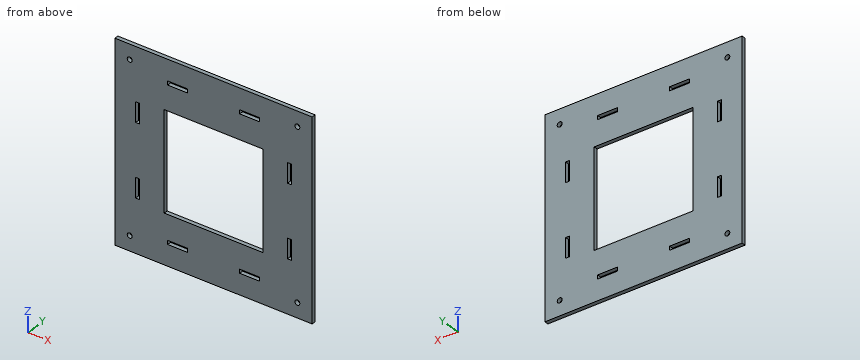
from build123d import *

# Parameters (mm, degrees)
CROQUIS1_W              = 200
CROQUIS1_H              = 200
CROQUIS1_R              = 2.5
SALIENTE_EXTRUIR1_DEPTH = 4
CROQUIS2_W              = 150
CROQUIS2_H              = 150
CROQUIS2_W_2            = 4
CROQUIS2_H_2            = 20
CROQUIS2_W_3            = 20
CROQUIS2_H_3            = 4
CORTAR_EXTRUIR1_DEPTH   = 4
CROQUIS3_W              = 150
CROQUIS3_H              = 150
CROQUIS3_W_2            = 100
CROQUIS3_H_2            = 100
SALIENTE_EXTRUIR2_DEPTH = 4


with BuildPart() as part:
    # Croquis1 → Saliente-Extruir1 (new body)
    with BuildSketch(Plane(origin=(0, 0, 0), x_dir=(1, 0, 0), z_dir=(0, 1, 0))):
        with Locations((100, 100)):
            Rectangle(CROQUIS1_W, CROQUIS1_H)
        with Locations(Location((15, 185, 0), (0, 0, 270))):
            Circle(CROQUIS1_R, mode=Mode.SUBTRACT)
        with Locations(Location((185, 185, 0), (0, 0, 270))):
            Circle(CROQUIS1_R, mode=Mode.SUBTRACT)
        with Locations(Location((185, 15, 0), (0, 0, 270))):
            Circle(CROQUIS1_R, mode=Mode.SUBTRACT)
        with Locations(Location((15, 15, 0), (0, 0, 270))):
            Circle(CROQUIS1_R, mode=Mode.SUBTRACT)
    extrude(amount=SALIENTE_EXTRUIR1_DEPTH)

    # Croquis2 → Cortar-Extruir1 (cut)
    with BuildSketch(Plane(origin=(0, 4, 0), x_dir=(1, 0, 0), z_dir=(0, 1, 0))):
        with Locations((100, 100)):
            Rectangle(CROQUIS2_W, CROQUIS2_H)
        with Locations((23, 136.5)):
            Rectangle(CROQUIS2_W_2, CROQUIS2_H_2)
        with Locations((63.5, 177)):
            Rectangle(CROQUIS2_W_3, CROQUIS2_H_3)
        with Locations((177, 136.5)):
            Rectangle(CROQUIS2_W_2, CROQUIS2_H_2)
        with Locations((136.5, 177)):
            Rectangle(CROQUIS2_W_3, CROQUIS2_H_3)
        with Locations((136.5, 23)):
            Rectangle(CROQUIS2_W_3, CROQUIS2_H_3)
        with Locations((177, 63.5)):
            Rectangle(CROQUIS2_W_2, CROQUIS2_H_2)
        with Locations((23, 63.5)):
            Rectangle(CROQUIS2_W_2, CROQUIS2_H_2)
        with Locations((63.5, 23)):
            Rectangle(CROQUIS2_W_3, CROQUIS2_H_3)
    extrude(amount=-CORTAR_EXTRUIR1_DEPTH, mode=Mode.SUBTRACT)

    # Croquis3 → Saliente-Extruir2 (add)
    with BuildSketch(Plane(origin=(0, 4, 0), x_dir=(1, 0, 0), z_dir=(0, 1, 0))):
        with Locations((100, 100)):
            Rectangle(CROQUIS3_W, CROQUIS3_H)
        with Locations((100, 100)):
            Rectangle(CROQUIS3_W_2, CROQUIS3_H_2, mode=Mode.SUBTRACT)
    extrude(amount=-SALIENTE_EXTRUIR2_DEPTH)


solid = part.part
The listing builds one solid part. Answer for the finished solid, in the listing's coordinates (mm). Round coordinates to 2 decimals unless told otherwise and drop trailing zeros. Order: outer loops, then holes, each group sorted by start corner. A loop starts at its lowest first (then second) coordinate and runs counter-clockwise, first axis right, second up. Notation, with made-up numbers: (32, 2.5) -> (47, 2.5) arc R28 ccw to (47, 28.5) -> close; hole circle Ø5 at (-13, 10.5). An arc over 180 degrees is marked (long way). One line per item, written item: value.
Item 1: Find section A-A, the plane z = -185. Give the vertices of the cut face in (x, y).
Taken from the geometry:
outline: (0, 0) -> (12.5, 0) -> (12.5, 4) -> (0, 4) -> close; (17.5, 0) -> (182.5, 0) -> (182.5, 4) -> (17.5, 4) -> close; (187.5, 0) -> (200, 0) -> (200, 4) -> (187.5, 4) -> close
Item 2: Straight lines are drawn through the part: L1, parallel to X at y = 2.8, z = -15; L2, parallel to X at y = 2.55, z = -176.5; L3, parallel to X at y = 2.1, z = -140. For each, find the intervals that lie inside material, in ascending order.
Taken from the geometry:
L1: x = 0 to 12.5, 17.5 to 182.5, 187.5 to 200
L2: x = 0 to 53.5, 73.5 to 126.5, 146.5 to 200
L3: x = 0 to 21, 25 to 50, 150 to 175, 179 to 200
Item 3: Find section C-C, the plane z = -124. Give the vertices of the cut face in (x, y), then the cut area to 3 significant figures.
Taken from the geometry:
outline: (0, 0) -> (50, 0) -> (50, 4) -> (0, 4) -> close; (150, 0) -> (200, 0) -> (200, 4) -> (150, 4) -> close
area: 400 mm2
Item 4: Find section D-D, the plane x = 15. Give the vertices of the cut face in (y, z).
Taken from the geometry:
outline: (0, -200) -> (4, -200) -> (4, -187.5) -> (0, -187.5) -> close; (0, -182.5) -> (4, -182.5) -> (4, -17.5) -> (0, -17.5) -> close; (0, -12.5) -> (4, -12.5) -> (4, 0) -> (0, 0) -> close
Item 5: Given P1, Ø3, axis at x = 15, z = -15, coming from the +Y side, flat-ended and moving along its own axis, determine where the tip first touches the part or whether it passes through.
Taken from the geometry:
P1: passes through
Item 6: Find section B-B, the plane x = 122. Give the vertices of the cut face in (y, z), then the cut area to 3 significant figures.
Taken from the geometry:
outline: (0, -200) -> (4, -200) -> (4, -150) -> (0, -150) -> close; (0, -50) -> (4, -50) -> (4, 0) -> (0, 0) -> close
area: 400 mm2
